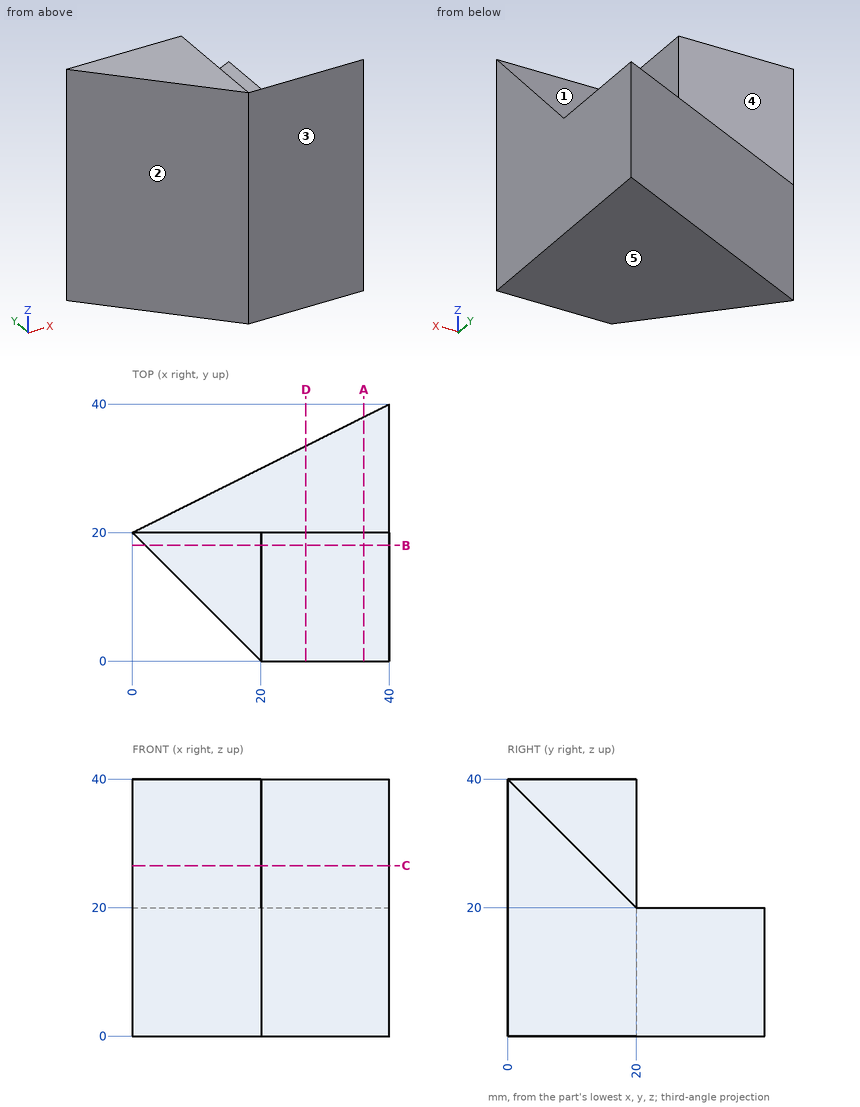
The drawing under review shows one solid part. Ordinate dimensions are in mm from its lowest x, y, z. A direction names the side the tool comes from. Give positions to 0.01 mm unless a question says otherwise; leave off trailing zeros. Write each loop counter-clockwise with the first axis right and the second up, starting at its lowest first coordinate (ties: lowest second). Pieces come first, ordered by that corner, then holes. Notation, with made-up numbers: (26.25, 57.5) - (64.25, 57.5) arc R11 ccw to (64.25, 71.5) - close; hole circle Ø10 at (2, -5.5). An arc over 180 degrees is marked (long way). Answer in a Markdown table with one row per item. Add a question column.
1. We need section C-C on z = 26.5. Write out the cut boundary in (x, y).
2. Draft analysis for pull direction Y (two halves, no side actions). For the marked faces 3, 4 and 5, state which applies: +Y half, -Y half, draft (parallel to the pull), parting line (faces both ways), or undercut.
3. We need section A-A on x = 36. Write out the cut boundary in (y, z), then the cut area to 3 significant figures.
4. Wall thickness on line 1 along Z through (x, y) = (35, 25); line 2 along Y through (x, z) = (15, 14.5); line 3 along X through (y, z) = (21.5, 17): over which ranges is each line inside the solid? List them lowest first. Write a range as [from, to].
5. Tool access review of the marked faces 1 and 2: name each direction out of +Z, -Z, +X, -X, +Y, -Y from which nothing blocks a thin tool from reaching the whole face with its end or side.
6. Insertion check: P1, Ø6, axis at x = 26, y = 21.5, coming from the -Z side; P2, Ø6, axis at x = 6, z = 30, coming from the +Y side; P3, Ø1.5, axis at x = 23, z = 32, coming from the +Y side; P4, Ø16, axis at x = 28.5, y = 30, coming from the +Z side. Each pin has a flat end and moves straight along its axis. Give the tip position at first contact, or say it passes through.
7. We need section B-B on y = 18. Write out the cut boundary in (x, z).
8. We need section D-D on x = 27. Write out the cut boundary in (y, z).
Ans:
| question | item | result |
|---|---|---|
| 1 | outline | (0, 20) - (20, 0) - (40, 0) - (40, 13.5) - (20, 13.5) - (20, 20) - close |
| 2 | face 3 | -Y half |
| 2 | face 4 | +Y half |
| 2 | face 5 | draft |
| 3 | outline | (0, 0) - (38, 0) - (38, 20) - (20, 20) - (0, 40) - close |
| 3 | area | 960 mm^2 |
| 4 | line 1 | z = [0, 20] |
| 4 | line 2 | y = [5, 27.5] |
| 4 | line 3 | x = [3, 40] |
| 5 | face 1 | +Z, +X, +Y |
| 5 | face 2 | +Z, -Z, -X, -Y |
| 6 | P1 | stops at z = 0 |
| 6 | P2 | stops at y = 20 |
| 6 | P3 | stops at y = 8.75 |
| 6 | P4 | stops at z = 20 |
| 7 | outline | (2, 0) - (40, 0) - (40, 22) - (20, 22) - (20, 40) - (2, 40) - close |
| 8 | outline | (0, 0) - (33.5, 0) - (33.5, 20) - (20, 20) - (0, 40) - close |
